```python
from build123d import *

# Parameters (mm, degrees)
F3_R     = 12.8249637965
F4_DEPTH = 30.4
F5_R     = 0.75
F6_DEPTH = 72


with BuildPart() as f1:
    # F0 (on Front) → F1 (revolve)
    with BuildSketch(Plane.XZ):
        with BuildLine():
            Line((0, 71.9589648982), (0, 71.956420194))
            Line((0, 71.956420194), (0, 43.3337725699))
            add(Edge.make_bspline(
                [(0, 43.3337725699), (0.6768933098, 42.5310779527), (1.4235595832, 41.9677112034), (2.2170609058, 41.6128150429)],
                knots=[0, 0, 0, 0, 0.0466672624, 0.0466672624, 0.0466672624, 0.0466672624], degree=3))
            add(Edge.make_bspline(
                [(2.2170609058, 41.6128150429), (7.914921835, 39.0644273981), (24.8773683832, 56.2108187873), (11.8622883606, 75.4374940312), (0.0647357854, 72.0839224676), (0, 71.9589648982)],
                knots=[0.0466672624, 0.0466672624, 0.0466672624, 0.0466672624, 0.3817688732, 0.747309423, 0.9958359163, 0.9958359163, 0.9958359163, 0.9958359163], degree=3))
        make_face()
        with BuildLine():
            add(Edge.make_bspline(
                [(0, 43.3337725699), (0.6768933098, 42.5310779527), (1.4235595832, 41.9677112034), (2.2170609058, 41.6128150429)],
                knots=[0, 0, 0, 0, 0.0466672624, 0.0466672624, 0.0466672624, 0.0466672624], degree=3))
            Line((0, 43.3337725699), (0, -43.0109836161))
            add(Edge.make_bspline(
                [(0, -43.0109836161), (1.9403692446, -43.4574948657), (4.6873576342, -42.6522625523), (7.8571672052, -44.4734265141), (10.8356003842, -38.8294957891), (16.3980803441, -13.1165207328), (18.7361219996, 16.8001032293), (4.7362580885, 18.8698801439), (2.3664417141, 19.0885338353), (2.2170609058, 18.8893601298)],
                knots=[0, 0, 0, 0, 0.1006535168, 0.1744949217, 0.2698143913, 0.5106129914, 0.7495537831, 0.8979870835, 0.9616249414, 0.9616249414, 0.9616249414, 0.9616249414], degree=3))
            Line((2.2170609058, 18.8893601298), (2.2170609058, 41.6128150429))
        make_face()
    revolve(axis=Axis((0, 0, 16.7866609991), (0, 0, -1)))

    # F3 (on offset) → F4 (cut)
    with BuildSketch(Plane.XY.offset(76.3)):
        Circle(F3_R)
    extrude(amount=-F4_DEPTH, mode=Mode.SUBTRACT)

    # F5 (on Top) → F6 (cut)
    with BuildSketch(Plane.XY):
        Circle(F5_R)
    extrude(amount=F6_DEPTH, mode=Mode.SUBTRACT)


solid = f1.part
```
The listing builds one solid part. Answer for the finished solid, in the listing's coordinates (mm). A direction names the side the tool comes from. Round coordinates to 2 decimals unless told otherwise and drop trailing zeros.
1) For faces 1 (the face through (12.233, 3.852, 58.285)), 2 (the face through (-0.481, 2.164, 30.41)), determine the directions among +Z, -Z, +X, -X, +Y, -Y from which every point of the face is accessible in a straight line to the end or side of a thin tool.
Outcome:
face 1: +Z
face 2: none
2) Consider line 1 (X direction, y = 0, z = 32.5); line 2 (Y direction, x = 0, z = 56.5). Determine where each line is inside the solid, lowest interval first.
Outcome:
line 1: x = -2.22 to -0.75, 0.75 to 2.22
line 2: y = -18.42 to -12.82, 12.82 to 18.42
3) Given P1, Ø8, axis at y = -9.5, z = 6, coming from the +X side; P2, Ø7.5, axis at x = -3.5, y = 5, coming from the +Z side; P3, Ø1.4, axis at x = 0, y = 0, coming from the -Z side, each flat-ended and moving along its own axis, determine where each tip first touches the part or whether it passes through.
Outcome:
P1: stops at x = 15.98
P2: stops at z = 45.9
P3: stops at z = -43.14
